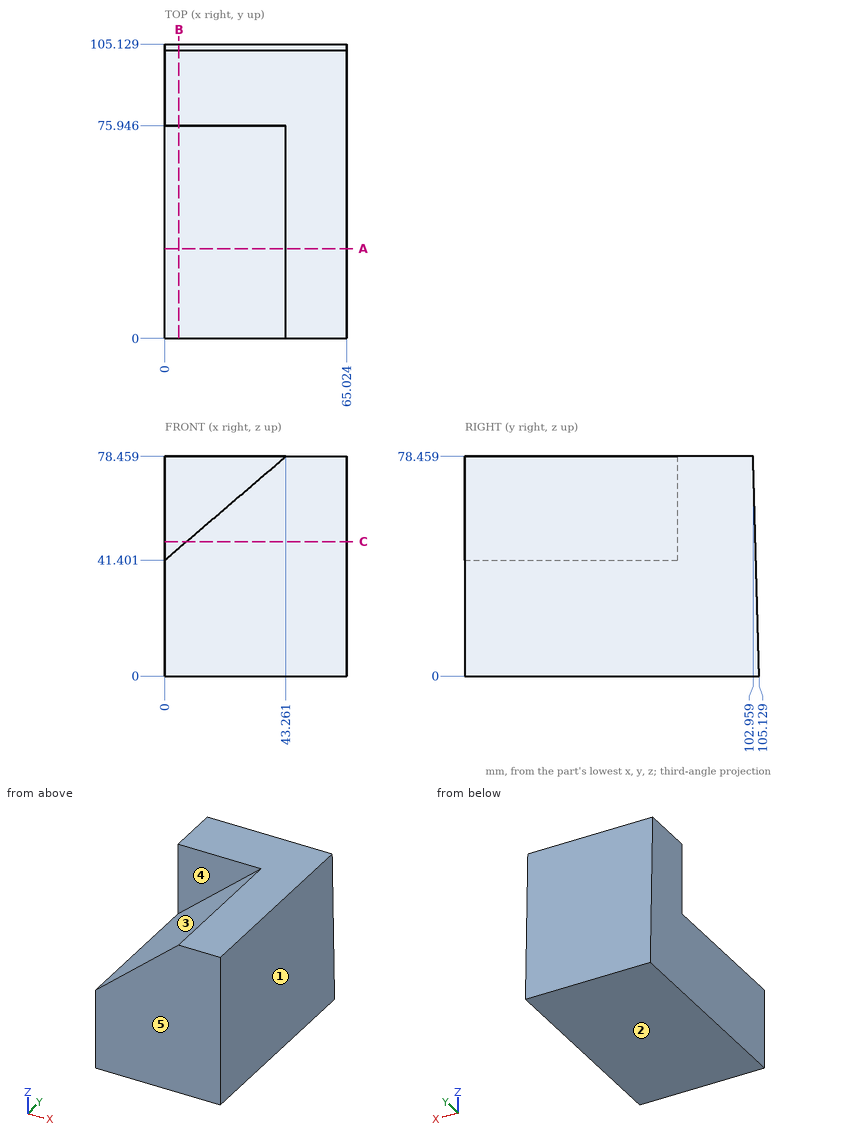
The figure shows three views and two pictorial views of one solid part (mm, origin at its lowest corner). Answer the questions. A direction names the side the tool comes from. Coordinates: 2 decimals unless noted, no trailing zeros. Loops run counter-clockwise (first coordinate to the right, second up) from the corner with the lowest first, then second, coordinate; pieces in that order, holes last. Notation, with made-up numbers: (-16.5, -38) -> (15.5, -38) arc R23 cw to (15.5, -28) -> close; hole circle Ø3 at (37, 61). An arc over 180 degrees is marked (long way). Return JSON: item names as keys, results as strings. Group by question number.
(1) Which of the six approach directions +Z, -Z, +X, -X, +Y, -Y give full straight-line access (tool end or side, diameter ignored) to the marked faces 4 and 5?
(2) Determine the mould class of the marked faces 1, 2 and 3 for opening direction X: released by +X, released by -X, zero draft, split by the parting line, or undercut.
(3) Find the intervals of material crossed by probe 1 along X at (y, z) = (23.5, 74.5) (1 decimal); probe 2 along Z at (x, y) = (42, 5.5); probe 3 along Y at (x, z) = (35.5, 30.5) (1 decimal), in increasing order. Write a range as from..to.
(4) A cutting plane is placed at C-C on z = 48. Write down the section's boundary in (x, y).
(5) Given pin 1 Ø1.5 at (x, z) = (23.5, 44.5) entering from +Y; pin 2 Ø1.5 at (y, z) = (42.5, 64) entering from -X (1 decimal); pin 3 Ø12 at (x, z) = (57.5, 8.5) entering from +Y, each flat-ended and moving along its own axis, determine where each tip first touches the part or whether it passes through.
(6) A cutting plane is placed at B-B on x = 5. Write down the section's boundary in (y, z).
(7) A cutting plane is placed at A-A on y = 32. Write down the section's boundary in (x, z).
The answers:
{
 "1": {"face 4": "+Z, -X, -Y", "face 5": "+Z, -Z, +X, -X, -Y"},
 "2": {"face 1": "released by +X", "face 2": "zero draft", "face 3": "released by -X"},
 "3": {"probe 1": "x = 38.6..65", "probe 2": "z = 0..77.38", "probe 3": "y = 0..104.3"},
 "4": {"outline": "(0, 75.95) -> (7.7, 75.95) -> (7.7, 0) -> (65.02, 0) -> (65.02, 103.8) -> (0, 103.8) -> close"},
 "5": {"pin 1": "stops at y = 103.92", "pin 2": "stops at x = 25.5", "pin 3": "stops at y = 105.06"},
 "6": {"outline": "(0, 0) -> (105.13, 0) -> (102.96, 78.46) -> (75.95, 78.46) -> (75.95, 45.68) -> (0, 45.68) -> close"},
 "7": {"outline": "(0, 0) -> (65.02, 0) -> (65.02, 78.46) -> (43.26, 78.46) -> (0, 41.4) -> close"}
}
